```python
from build123d import *

# Parameters (mm, degrees)
ESQUISSE2_R             = 2
BOSS_EXTRU_1_DEPTH      = 5
ESQUISSE3_R             = 1.5
BOSS_EXTRU_2_DEPTH      = 5
ESQUISSE5_R             = 17.5
ENL_V_MAT_EXTRU_1_DEPTH = 68.566633777
ESQUISSE7_R             = 19.5
ESQUISSE8_R             = 12
CONG_2_R                = 2


with BuildPart() as part:
    # Esquisse2 → Boss.-Extru.1 (new body)
    with BuildSketch(Plane(origin=(0, 0, 0), x_dir=(1, 0, 0), z_dir=(0, 1, 0))):
        Polygon((5, -19.739092363), (27.5, -19.739092363), (27.5, -11.739092363), (-27.5, -11.739092363), (-27.5, -19.739092363), (-5, -19.739092363), (-5, -39.739092363), (5, -39.739092363), align=None)
        with Locations(Location((-21.5, -15.739092363, 0), (0, 0, 270))):
            Circle(ESQUISSE2_R, mode=Mode.SUBTRACT)
        with Locations(Location((21.5, -15.739092363, 0), (0, 0, 270))):
            Circle(ESQUISSE2_R, mode=Mode.SUBTRACT)
    extrude(amount=BOSS_EXTRU_1_DEPTH)

    # Esquisse3 → Boss.-Extru.2 (add)
    with BuildSketch(Plane.XY.offset(39.739092363)):
        Polygon((-5, 5), (5, 5), (5, -15), (20, -15), (20, -55), (-20, -55), (-20, -15), (-5, -15), align=None)
        with Locations((-17.5, -17.5)):
            Circle(ESQUISSE3_R, mode=Mode.SUBTRACT)
        with Locations((17.5, -17.5)):
            Circle(ESQUISSE3_R, mode=Mode.SUBTRACT)
        with Locations((17.5, -52.5)):
            Circle(ESQUISSE3_R, mode=Mode.SUBTRACT)
        with Locations((-17.5, -52.5)):
            Circle(ESQUISSE3_R, mode=Mode.SUBTRACT)
    extrude(amount=BOSS_EXTRU_2_DEPTH)

    # Esquisse5 → Enlèv. mat.-Extru.1 (cut, through all)
    with BuildSketch(Plane(origin=(0, 0, 39.739092363), x_dir=(-1, 0, 0), z_dir=(0, 0, -1))):
        with Locations((0, -35)):
            Circle(ESQUISSE5_R)
    extrude(amount=-ENL_V_MAT_EXTRU_1_DEPTH, mode=Mode.SUBTRACT)

    # Esquisse7 → Lissage3 section 0
    with BuildSketch(Plane(origin=(0, 0, 39.739092363), x_dir=(-1, 0, 0), z_dir=(0, 0, -1))):
        with Locations((0, -35)):
            Circle(ESQUISSE7_R)
    # Esquisse8 → Lissage3 section 1
    with BuildSketch(Plane(origin=(0, 0, 19.739092363), x_dir=(-1, 0, 0), z_dir=(0, 0, -1))):
        with Locations((0, -35)):
            Circle(ESQUISSE8_R)
    loft()

    # Enlèvement de matière-Lissage1: read off the stored shape, not the designer's step
    # Enlèvement de matière-Lissage1: loft between two sections, ruled curve by curve
    enl_vement_de_mati_re_lissage1_from = [
        Edge.make_bspline([(16.003401512, -27.918959112, 39.739092363), (30.165483288, -59.925762135, 39.739092363), (-1.841319736, -74.087843911, 39.739092363), (-16.003401512, -42.081040888, 39.739092363), (-30.165483288, -10.074237865, 39.739092363), (1.841319736, 4.087843911, 39.739092363), (16.003401512, -27.918959112, 39.739092363)], [0, 0, 0, 0, 0.5, 0.5, 0.5, 1, 1, 1, 1], 3, [1, 0.333333333, 0.333333333, 1, 0.333333333, 0.333333333, 1]),
    ]
    enl_vement_de_mati_re_lissage1_to = [
        Edge.make_bspline([(7.154976715, -28.013848827, 19.739092363), (21.127279061, -42.323802256, 19.739092363), (6.817325632, -56.296104602, 19.739092363), (-7.154976715, -41.986151173, 19.739092363), (-21.127279061, -27.676197744, 19.739092363), (-6.817325632, -13.703895398, 19.739092363), (7.154976715, -28.013848827, 19.739092363)], [0, 0, 0, 0, 0.5, 0.5, 0.5, 1, 1, 1, 1], 3, [1, 0.333333333, 0.333333333, 1, 0.333333333, 0.333333333, 1]),
    ]
    enl_vement_de_mati_re_lissage1 = Solid(Shell([*[Face.make_surface_from_curves(enl_vement_de_mati_re_lissage1_from[k], enl_vement_de_mati_re_lissage1_to[k]) for k in range(1)], Face(Wire(enl_vement_de_mati_re_lissage1_from)), Face(Wire(enl_vement_de_mati_re_lissage1_to))]))
    add(enl_vement_de_mati_re_lissage1, mode=Mode.SUBTRACT)

    # Congé2
    cong_2_edges = [part.edges().sort_by_distance(p)[0] for p in [
        (-20, -15, 42.239092363),
        (-20, -55, 42.239092363),
        (20, -55, 42.239092363),
        (20, -15, 42.239092363),
        (-5, 5, 32.239092363),
        (5, 5, 32.239092363),
        (5, -15, 42.239092363),
        (-5, -15, 42.239092363),
        (-16.25, 5, 19.739092363),
        (16.25, 5, 19.739092363),
        (0, 5, 44.739092363),
        (27.5, 2.5, 19.739092363),
        (-27.5, 2.5, 19.739092363),
        (-5, 2.5, 19.739092363),
        (5, 2.5, 19.739092363),
        (0, 0, 39.739092363),
    ]]
    fillet(cong_2_edges, radius=CONG_2_R - 0.0001)  # a hair under: the kernel refuses the full size


solid = part.part
```
Here's how the part is built. I have some questions about the finished solid (model axes, mm). A direction names the side the tool comes from. Round coordinates to 2 decimals unless told otherwise and drop trailing zeros. Order: outer loops, then holes, each group sorted by start corner. A loop starts at its lowest first (then second) coordinate and runs counter-clockwise, first axis right, second up. Notation, with made-up numbers: (-40, -20) -> (-17, -20) arc R26 cw to (-17, 10) -> close; hole circle Ø1 at (13, -11.5). An arc over 180 degrees is marked (long way). Use a Markdown table: item, result. Add a question column.
(1) Suppose I cut it at C-C, the plane z = 24.5. Count the separate pieces of the cut face and the enclosed holes in it, and give its area (3 significant figures).
(2) Suppose I cut it at B-B, the plane z = 42. Please give me the cut outline in (x, y).
(3) For pin 1 Ø2.5 at (x, y) = (-17.5, -52.5) entering from -Z; pin 2 Ø10 at (y, z) = (-40.5, 34.5) entering from +X; pin 3 Ø5 at (x, z) = (21.5, 15.74) entering from -Y; pin 4 Ø2.5 at (y, z) = (-32, 43) entering from -X, each with a flat end and sliding along its axis, tell me the tip position at first contact or that it passes through.
(4) I need wall thicknesses on line 1 along Y through (x, z) = (2.5, 25); line 2 along X through (y, z) = (-35, 43.75); line 3 along Y through (x, z) = (-4, 21.5). Which ranges of each line are inside material? Lowest first, please.
(5) If we mould it in two halves opening along Y, with no side actions, what happens to faces 4 (the face through (0, -55, 42)), 5 (the face through (20.734, 2.465, 17.587)), 6 (the face through (4.43, 4.4, 33.08)), 7 (the face through (0, 0, 19))? For each: released by +Y, released by -Y, zero draft, split by the parting line, or undercut.
(6) For faces 1 (the face through (-13, -15, 42)), 2 (the face through (0.07, -0.6, 39.17)), 3 (the face through (0, -15, 39.739)), which set-ups out of +Z, -Z, +X, -X, +Y, -Y let a thin tool reach every point of the face, with its end or its side?
Verdict:
| question | item | result |
|---|---|---|
| 1 | separate pieces | 2 |
| 1 | enclosed holes | 1 |
| 1 | area | 222 mm2 |
| 2 | outline | (-20, -53) arc R2 ccw to (-18, -55) -> (18, -55) arc R2 ccw to (20, -53) -> (20, -17) arc R2 ccw to (18, -15) -> (7, -15) arc R2 cw to (5, -13) -> (5, 3) arc R2 ccw to (3, 5) -> (-3, 5) arc R2 ccw to (-5, 3) -> (-5, -13) arc R2 cw to (-7, -15) -> (-18, -15) arc R2 ccw to (-20, -17) -> close; hole circle Ø3 at (-17.5, -52.5); hole circle Ø3 at (-17.5, -17.5); hole circle Ø35 at (0, -35); hole circle Ø3 at (17.5, -52.5); hole circle Ø3 at (17.5, -17.5) |
| 3 | pin 1 | through |
| 3 | pin 2 | x = 18.93 |
| 3 | pin 3 | y = 0 |
| 3 | pin 4 | x = -20 |
| 4 | line 1 | -48.75 to -46.52, -23.48 to -21.25, 0 to 5 |
| 4 | line 2 | -20 to -17.5, 17.5 to 20 |
| 4 | line 3 | -47.01 to -44.79, -25.21 to -22.99, 0 to 4.74 |
| 5 | face 4 | released by -Y |
| 5 | face 5 | zero draft |
| 5 | face 6 | released by +Y |
| 5 | face 7 | undercut |
| 6 | face 1 | +Z, -Z, -X, +Y |
| 6 | face 2 | -Z, +X, -X |
| 6 | face 3 | -Z |
